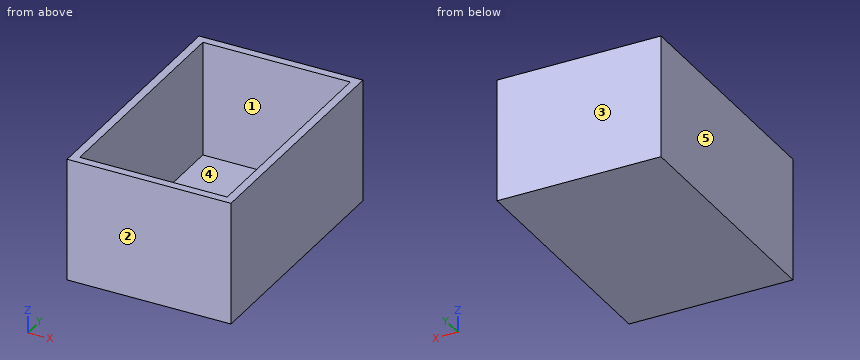
Autodesk Inventor part; units mm, degrees
ref_plane "Work Plane1" through (0, -300, -150) normal (0, 0, -1) x (-1, 0, 0)
ref_plane "YZ Plane" through (0, 0, 0) normal (1, 0, 0) x (0, 1, 0)
ref_plane "XZ Plane" through (0, 0, 0) normal (0, 1, 0) x (-1, 0, 0)
sketch "Sketch1" plane through (0, 0, 0) normal (1, 0, 0) x (0, 1, 0)
  line L0 (0, 0) -> (-300, 0)
  line L1 (-300, 0) -> (-300, -150)
  line L2 (-300, -150) -> (0, -150)
  line L3 (0, -150) -> (0, 0)
  dimension "d0" = 300
  dimension "d1" = 150
extrude "Extrusion1" add sketch "Sketch1" along normal blind 200
sketch "Sketch2" plane through (0, 0, 0) normal (-1, 0, 0) x (0, 0, 1)
  point P0 (0, 0)
sketch "Sketch3" plane through (0, -300, 0) normal (0, 0, 1) x (1, 0, 0)
  point P0 (0, 300)
sketch "Sketch4" plane through (0, -300, 0) normal (0, 0, 1) x (1, 0, 0)
  point P0 (0, 300)
sketch "Sketch5" plane through (0, -300, 0) normal (0, 0, 1) x (1, 0, 0)
  line L0 (0, 0) -> (200, 0)
  line L1 (0, 0) -> (190, 0)
  line L2 (190, 10) -> (190, 290)
  line L3 (190, 290) -> (0, 290)
  line L4 (0, 10) -> (0, 0)
  line L5 (-111.4723, 0) -> (-111.4723, 10)
  line L6 (10, 10) -> (190, 10)
  line L7 (0, -40.6594) -> (10, -40.6594)
  line L8 (10, 0) -> (10, 290)
  point P0 (0, 300)
  dimension "d4" = 190
  dimension "d5" = 290
  dimension "d6" = 10
  dimension "d7" = 10
extrude "Extrusion2" cut sketch "Sketch5" against normal blind 140
ref_plane "Work Plane1" through (0, -300, -150) normal (0, 0, -1) x (-1, 0, 0)
sketch "Sketch6" plane through (0, -300, -150) normal (0, 0, -1) x (-1, 0, 0)
  point P0 (0, 300)
sketch "Sketch7" plane through (0, -300, -150) normal (0, 0, -1) x (-1, 0, 0)
  line L0 (0, 340.13) -> (-50, 340.13)
  line L1 (-50, 340.13) -> (-50, -164.6167)
  line L2 (0, 300) -> (-200, 300)
  line L3 (0, 300) -> (0, 225)
  line L4 (0, 0) -> (0, 300)
  line L5 (-50, 225) -> (-50, 275)
  line L6 (-50, 275) -> (-70, 275)
  line L7 (-70, 275) -> (-70, 175)
  line L8 (-70, 175) -> (-30, 175)
  line L9 (-30, 175) -> (-30, 275)
  line L10 (-30, 275) -> (-50, 275)
  dimension "d14" = 50
  dimension "d15" = 75
  dimension "d16" = 50
  dimension "d17" = 20
  dimension "d18" = 100
  dimension "d19" = 40
  dimension "d20" = 100
  dimension "d21" = 20
extrude "Extrusion3" cut sketch "Sketch7" against normal blind 50
sketch "Sketch8" plane through (0, -300, -150) normal (0, 0, -1) x (-1, 0, 0)
  line L0 (0, 0) -> (0, 300)
  line L1 (0, 0) -> (0, 75)
  line L2 (-54.3985, -5.8801) -> (-4.3985, -5.8801)
  line L3 (0, 0) -> (-200, 0)
  line L4 (-100, 0) -> (-100, 75)
  line L5 (-54.3985, 75) -> (-34.3985, 75)
  line L6 (-34.3985, 75) -> (-34.3985, 25)
  line L7 (-34.3985, 25) -> (-74.3985, 25)
  line L8 (-74.3985, 25) -> (-74.3985, 125)
  line L9 (-74.3985, 125) -> (-34.3985, 125)
  line L10 (-34.3985, 125) -> (-34.3985, 75)
  line L11 (-10, 10) -> (-10, 290)
  line L12 (-200, 0) -> (-200, 300)
  line L13 (-200, 300) -> (-150, 300)
  line L14 (0, 300) -> (-200, 300)
  line L15 (-200, 300) -> (-200, 225)
  line L16 (-150, 225) -> (-170, 225)
  line L17 (-170, 225) -> (-170, 175)
  line L18 (-170, 175) -> (-130, 175)
  line L19 (-130, 175) -> (-130, 275)
  line L20 (-130, 275) -> (-170, 275)
  line L21 (-170, 275) -> (-170, 225)
  line L22 (-200, 0) -> (-200, 110.9429)
  line L23 (-200, 0) -> (-200, 75)
  line L24 (-200, 0) -> (-150, 0)
  line L25 (-150, 75) -> (-130, 75)
  line L26 (-130, 75) -> (-130, 25)
  line L27 (-130, 25) -> (-170, 25)
  line L28 (-170, 25) -> (-170, 125)
  line L29 (-170, 125) -> (-130, 125)
  line L30 (-130, 125) -> (-130, 75)
  dimension "d24" = 75
  dimension "d25" = 50
  dimension "d26" = 75
  dimension "d27" = 20
  dimension "d28" = 50
  dimension "d29" = 40
  dimension "d30" = 100
  dimension "d31" = 40
  dimension "d32" = 50
  dimension "d33" = 50
  dimension "d34" = 75
  dimension "d35" = 20
  dimension "d36" = 50
  dimension "d37" = 40
  dimension "d38" = 100
  dimension "d39" = 40
  dimension "d40" = 50
  dimension "d41" = 75
  dimension "d42" = 50
  dimension "d43" = 20
  dimension "d44" = 50
  dimension "d45" = 40
  dimension "d46" = 100
  dimension "d47" = 40
  dimension "d48" = 50
extrude "Extrusion4" cut sketch "Sketch8" against normal blind 50 contours L6 L7 L8 L9 L10 | L21 L20 L19 L18 L17 | L26 L27 L28 L29 L30
sketch "Sketch9" plane through (0, -300, -150) normal (0, 0, -1) x (-1, 0, 0)
  point P0 (0, 300)
sketch "Sketch14" plane through (0, -300, -150) normal (0, 0, -1) x (-1, 0, 0)
  line L0 (-30, 275) -> (-30, 175)
  line L1 (-70, 275) -> (-30, 275)
  line L2 (-30, 275) -> (-70, 275)
  line L3 (-70, 275) -> (-70, 175)
  line L4 (-30, 175) -> (-70, 175)
  line L5 (-70, 175) -> (-30, 175)
  line L6 (-30, 175) -> (-30, 275)
  line L7 (-130, 275) -> (-170, 275)
  line L8 (-130, 275) -> (-170, 275)
  line L9 (-170, 275) -> (-170, 175)
  line L10 (-170, 275) -> (-170, 175)
  line L11 (-130, 275) -> (-130, 175)
  line L12 (-170, 175) -> (-130, 175)
  line L13 (-130, 175) -> (-130, 275)
  line L14 (-34.3985, 25) -> (-34.3985, 125)
  line L15 (-74.3985, 25) -> (-74.3985, 125)
  line L16 (-34.3985, 125) -> (-74.3985, 125)
  line L17 (-74.3985, 125) -> (-74.3985, 25)
  line L18 (-34.3985, 25) -> (-74.3985, 25)
  line L19 (-74.3985, 25) -> (-34.3985, 25)
  line L20 (-34.3985, 25) -> (-34.3985, 125)
  line L21 (-130, 125) -> (-170, 125)
  line L22 (-130, 125) -> (-170, 125)
  line L23 (-130, 25) -> (-170, 25)
  line L24 (-170, 125) -> (-170, 25)
  line L25 (-170, 25) -> (-130, 25)
  line L26 (-130, 25) -> (-130, 125)
  point P0 (0, 300)
  dimension "d52" = 100
extrude "Extrusion5" add sketch "Sketch14" against normal blind 10
Input: part model. Units: mm. Frame: model coordinates. Face numbers are marked on the shaded views. A direction names the side the tool comes from. Give positions to 0.01 mm unless a question says otherwise; leave off trailing zeros. Write each loop counter-clockwise with the first axis right and the second up, starting at its lowest first coordinate (ties: lowest second). Pieces come first, ordered by that corner, then holes.
Q1. Set-up query: the marked faces 1 and 2. Return all of +Z, -Z, +X, -X, +Y, -Y with unobstructed straight access to the full face (end or side cutting, diameter ignored); none if empty.
Q2. Pull-direction query (X, two-part tool) for the marked faces 3, 4 and 5; classes: pulls with the +X half, pulls with the -X half, needs draft (parallel to the pull), parting line crosses it, or undercut.
Q3. Section B-B, the plane y = -92. Output: boundary loops of the cut face in (x, z).
Q4. Material intervals for probe 1 along Y at (x, z) = (83, -91); probe 2 along X at (y, z) = (-41, -61.5); probe 3 along Z at (x, y) = (62, -276.5), sorted ascending.
Q5. Section A-A, the plane z = -29.5. Output: boundary loops of the cut face in (x, y), plus the area to 3 significant figures.
Q6. Section C-C, the plane x = 59.5. Output: boundary loops of the cut face in (y, z).
Q7. First-contact query: P1, Ø2, axis at x = 155, y = -38, coming from the +Z side. Flat tip, straight axial feed; report the tip coordinate or a pass-through.
Filled in:
1. face 1: +Z
1. face 2: +Z, -Z, +X, -X, -Y
2. face 3: needs draft
2. face 4: undercut
2. face 5: pulls with the -X half
3. outline: (0, -150) - (200, -150) - (200, 0) - (190, 0) - (190, -140) - (10, -140) - (10, 0) - (0, 0) - close
4. probe 1: y = -300 to -290, -10 to 0
4. probe 2: x = 0 to 10, 190 to 200
4. probe 3: z = -150 to -140
5. outline: (0, -300) - (200, -300) - (200, 0) - (0, 0) - close; hole (10, -290) - (190, -290) - (190, -10) - (10, -10) - close
5. area: 9,600 mm2
6. outline: (-300, -150) - (0, -150) - (0, 0) - (-10, 0) - (-10, -140) - (-290, -140) - (-290, 0) - (-300, 0) - close
7. P1: stops at z = -140
